For this review, take the finished solid that the model builds, in its own axes (mm). A direction names the side the tool comes from. Round coordinates to 2 decimals unless told otherwise and drop trailing zeros. Write each loop counter-clockwise with the first axis right and the second up, starting at its lowest first coordinate (ties: lowest second). Pieces come first, ordered by that corner, then holes.
from build123d import *

# Parameters (mm, degrees)
BOSS_EXTRUDE1_DEPTH = 2
SKETCH3_R           = 2.5
CUT_EXTRUDE1_DEPTH  = 2
BOSS_EXTRUDE2_DEPTH = 5
FILLET2_R           = 2
SKETCH8_R           = 3.8
SKETCH8_R_2         = 2.5
BOSS_EXTRUDE3_DEPTH = 1.2
SKETCH7_R           = 0.5000000000000009
CUT_EXTRUDE3_DEPTH  = 2
SKETCH15_R          = 0.5000000000000009
CUT_EXTRUDE5_DEPTH  = 3
SKETCH18_W          = 7
SKETCH18_H          = 7.573769237451616
BOSS_EXTRUDE4_DEPTH = 5
SKETCH19_R          = 0.9999999999999996
CUT_EXTRUDE6_DEPTH  = 3
SKETCH20_W          = 4.499999999999998
SKETCH20_H          = 4.5
CUT_EXTRUDE7_DEPTH  = 5


with BuildPart() as part:
    # Sketch2 → Boss-Extrude1 (new body)
    with BuildSketch(Plane.XY):
        with BuildLine():
            Line((0, 5.000000000000001), (-2.5, 6))
            Line((-2.5, 6), (-19.499999999999996, 5.999999999999998))
            Line((-19.499999999999996, 5.999999999999998), (-19.499999999999996, -4.000000000000002))
            Line((-19.499999999999996, -4.000000000000002), (-5.4999999999999964, -4.999999999999999))
            Line((-5.4999999999999964, -4.999999999999999), (-2.999999999999996, -4.0000000000000036))
            ThreePointArc((-2.999999999999996, -4.0000000000000036), (4.743416490252571, -1.5811388300841875), (0, 5.000000000000001))
        make_face()
    extrude(amount=BOSS_EXTRUDE1_DEPTH)

    # Sketch3 → Cut-Extrude1 (cut)
    with BuildSketch(Plane(origin=(0, 0, 0), x_dir=(-1, 0, 0), z_dir=(0, 0, -1))):
        Circle(SKETCH3_R)
    extrude(amount=-CUT_EXTRUDE1_DEPTH, mode=Mode.SUBTRACT)

    # Sketch4 → Boss-Extrude2 (add)
    with BuildSketch(Plane.XY.offset(2)):
        Polygon((-19.499999999999996, -4.000000000000002), (-19.499999999999996, 5.999999999999998), (-2.5, 6), (-5.349362666614333, 4.499999999999999), (-18.299999999999997, 4.499999999999997), (-18.299999999999997, -2.581892623469482), (-6.7590791740868275, -3.4062441110347046), (-5.4999999999999964, -4.999999999999999), (-19.292624540521615, -4.014812532819887), align=None)
    extrude(amount=BOSS_EXTRUDE2_DEPTH)

    # Fillet2
    fillet2_edges = [part.edges().sort_by_distance(p)[0] for p in [
        (-19.499999999999996, 0.9999999999999982, 0),
        (-19.499999999999996, 5.999999999999998, 3.5),
        (-12.499999999999996, -4.5, 0),
        (-10.999999999999998, 5.999999999999999, 0),
    ]]
    fillet(fillet2_edges, radius=FILLET2_R)

    # Sketch8 → Boss-Extrude3 (add)
    with BuildSketch(Plane.XY.offset(2)):
        Circle(SKETCH8_R)
        with Locations(Location((0, 0, 0), (0, 0, 180))):
            Circle(SKETCH8_R_2, mode=Mode.SUBTRACT)
    extrude(amount=BOSS_EXTRUDE3_DEPTH)

    # Sketch7 → Cut-Extrude3 (cut, along a direction that is not the sketch's normal)
    with BuildSketch(Plane.XZ.offset(-4.5)):
        with Locations((-10.349362666614333, 7)):
            Circle(SKETCH7_R)
    extrude(amount=-CUT_EXTRUDE3_DEPTH, dir=(0.6843021216730707, -0.7291986055072609, 0), mode=Mode.SUBTRACT)

    # Sketch15 → Cut-Extrude5 (cut, along a direction that is not the sketch's normal)
    with BuildSketch(Plane(origin=(-0.2763781559826011, -3.869294183756433, 0), x_dir=(0.9974586998307351, -0.07124704998790933, 0), z_dir=(0.07124704998790933, 0.9974586998307351, 0))):
        with Locations((-9.537755541479953, -7)):
            Circle(SKETCH15_R)
    extrude(amount=-CUT_EXTRUDE5_DEPTH, dir=(0.7271985173785733, 0.6864272112339407, 0), mode=Mode.SUBTRACT)

    # Sketch18 → Boss-Extrude4 (add)
    with BuildSketch(Plane.XY.offset(2)):
        with Locations((-14.799999999999997, 0.7131153812741895)):
            Rectangle(SKETCH18_W, SKETCH18_H)
    extrude(amount=BOSS_EXTRUDE4_DEPTH)

    # Sketch19 → Cut-Extrude6 (cut)
    with BuildSketch(Plane.XY.offset(6.999999999999999)):
        with Locations((-15.299999999999997, 0.9999999999999972)):
            Circle(SKETCH19_R)
    extrude(amount=-CUT_EXTRUDE6_DEPTH, mode=Mode.SUBTRACT)

    # Sketch20 → Cut-Extrude7 (cut)
    with BuildSketch(Plane.XY.offset(3.999999999999999)):
        with Locations((-15.299999999999997, 0.9999999999999969)):
            Rectangle(SKETCH20_W, SKETCH20_H)
    extrude(amount=-CUT_EXTRUDE7_DEPTH, mode=Mode.SUBTRACT)

    # Mirror1: part across plane


with BuildPart() as part_1:
    add(part.part)
    add(part.part.mirror(Plane.XY.offset(6.999999999999999)))


with BuildPart() as body_2:
    # Split1: the piece on the far side of the plane
    add(part_1.part)
    split(bisect_by=Plane.XY.offset(6.999999999999999), keep=Keep.BOTTOM)


with BuildPart() as part_2:
    add(part_1.part)

    # Split1
    split(bisect_by=Plane.XY.offset(6.999999999999999), keep=Keep.TOP)


solid = part_2.part
(1) Mouldability with a two-part tool opening along Y and no side actions: class faces 6 (the face through (-11.3, 1, 10)), 7 (the face through (-6, 0, 14)), 8 (the face through (-1, 5.4, 12.7)) as pulls with the +Y half, pulls with the -Y half, needs draft (parallel to the pull), parting line crosses it, or undercut.
Geometry check:
face 6: undercut
face 7: needs draft
face 8: pulls with the +Y half
(2) For faces 1 (the face through (-15, -1.25, 12)), 2 (the face through (-8, 4.5, 10)), 3 (the face through (-4, -4.4, 12.7)), 4 (the face through (-10, 6, 10)), 5 (the face through (-5, 1, 12)), list the 3-axis set-ups (+Z, -Z, +X, -X, +Y, -Y) from which the entire face can be reached by the end or side of a thin tool; tool diameter is ignored.
Geometry check:
face 1: +Z
face 2: -Z, +X
face 3: +Z, -Z, -Y
face 4: +Z, -Z, +X, -X, +Y
face 5: -Z
(3) We need section C-C, the plane y = -0.25. Give the boundary of the cut face in (x, z), and give its area (3 significant figures).
Geometry check:
outline: (-19.5, 7) - (-11.3, 7) - (-11.3, 12) - (-3.79, 12) - (-3.79, 10.8) - (-2.49, 10.8) - (-2.49, 14) - (-13.05, 14) - (-13.05, 10) - (-17.55, 10) - (-17.55, 14) arc R2 ccw to (-19.5, 12) - close; (2.49, 10.8) - (3.79, 10.8) - (3.79, 12) - (4.99, 12) - (4.99, 14) - (2.49, 14) - close
area: 64.3 mm2
(4) We need section D-D, the plane z = 12.75. Give the boundary of the cut face in (x, y).
Geometry check:
outline: (-19.35, -3.86) - (-5.19, -4.88) - (-3, -4) arc R5 ccw (long way) to (0, 5) - (-2.14, 5.85) - (-17.5, 5.85) arc R1.85 ccw to (-19.35, 4) - close; hole (-17.55, -1.25) - (-13.05, -1.25) - (-13.05, 3.25) - (-17.55, 3.25) - close; hole circle Ø5 at (0, 0)
(5) For line 1 along X through (y, z) = (-1, 12.5); line 2 along X through (y, z) = (0, 10.25); line 3 along Z through (x, y) = (-9.5, 1), list the stretches that pass through material, from the lowest coordinate up.
Geometry check:
line 1: x = -19.44 to -17.55, -13.05 to -2.29, 2.29 to 4.9
line 2: x = -19.5 to -17.55, -13.05 to -11.3
line 3: z = 12 to 14
(6) We need section B-B, the plane z = 9.75. Give the boundary of the cut face in (x, y), and give its area (3 significant figures).
Geometry check:
outline: (-19.5, -4) - (-5.5, -5) - (-6.76, -3.41) - (-11.41, -3.07) - (-11.3, -3.07) - (-11.3, 4.5) - (-5.35, 4.5) - (-2.5, 6) - (-17.5, 6) arc R2 ccw to (-19.5, 4) - close; hole circle Ø2 at (-15.3, 1)
area: 99.2 mm2
(7) For pin 1 Ø4 at (y, z) = (1, 9.5) entering from +X; pin 2 Ø1 at (x, y) = (-2.5, -4) entering from +Z; pin 3 Ø4 at (x, y) = (-6.5, 0) entering from -Z, all flat-tipped, find the tip position at first contact; note any pin that passes through.
Geometry check:
pin 1: stops at x = 3.8
pin 2: stops at z = 13.98
pin 3: stops at z = 12
(8) We need section A-A, the plane y = 1. Give the boundary of the cut face in (x, z).
Geometry check:
outline: (-19.5, 7) - (-16.3, 7) - (-16.3, 10) - (-17.55, 10) - (-17.55, 14) arc R2 ccw to (-19.5, 12) - close; (-14.3, 7) - (-11.3, 7) - (-11.3, 12) - (-3.67, 12) - (-3.67, 10.8) - (-2.29, 10.8) - (-2.29, 14) - (-13.05, 14) - (-13.05, 10) - (-14.3, 10) - close; (2.29, 10.8) - (3.67, 10.8) - (3.67, 12) - (4.9, 12) - (4.9, 14) - (2.29, 14) - close
